Model file for the job. Use its own axes, mm. Coordinates: 2 decimals unless noted, no trailing zeros. Write each loop counter-clockwise with the first axis right and the second up, starting at its lowest first coordinate (ties: lowest second). Pieces come first, ordered by that corner, then holes. Notation, with made-up numbers: M 51.5,-28.5 L 67.5,-28.5 A14 ccw 67.5,-14.5 Z; hole C 45.5,40.25 d3. An arc over 180 degrees is marked long. One line per question, with ' | ' between items. Start each with the question number.
(1) Cut at B-B (y = 1.5). Count the separate pieces of the cut face and the enclosed holes in it, plus the area to 3 significant figures.
(2) Two-plate mould, pull along Z, no slides. Class faces 1 (the face through (0.733, 1.479, 99.997)), 2 (the face through (42.495, 1.479, -41.232)), 3 (the face through (1, 3, 1)): +Z half, -Z half, draft (parallel to the pull), parting line (faces both ways), or undercut.
(3) Cut at A-A (x = 38). Write the cut outline in (y, z), plus the area to 3 significant figures.
(4) Wall check: probe 1 along Z at (x, y) = (-25, 2.15); probe 2 along Z at (x, y) = (-41, 1.8); probe 3 along X at (y, z) = (0.55, 91.5). Give the ranges that are in metal, low to high.
(5) Flat gauge pin, fed straight in: pin 1 Ø3.5 at (x, z) = (-42, 84.85) entering from -Y. Where does the tip first touch, or does it go through?
(6) Cut at D-D (x = -17.5). Write the cut outline in (y, z).
(7) Cut at C-C (x = -37.5). Write the cut outline in (y, z), plus the area to 3 significant figures.
Autodesk Inventor part; units mm, degrees
ref_plane "YZ Plane" through (0, 0, 0) normal (1, 0, 0) x (0, 1, 0)
ref_plane "XZ Plane" through (0, 0, 0) normal (0, 1, 0) x (-1, 0, 0)
ref_plane "XY Plane" through (0, 0, 0) normal (0, 0, 1) x (1, 0, 0)
sketch "Sketch1" plane through (0, 0, 0) normal (0, 1, 0) x (-1, 0, 0)
  line L0 (-50, 86.6025) -> (-50, -86.6025)
  line L1 (50, -86.6025) -> (50, 86.6025)
  arc A0 (50, 86.6025) -> (-50, 86.6025) centre (0, 0) ccw
  arc A1 (-50, -86.6025) -> (50, -86.6025) centre (0, 0) ccw
  circle A2 centre (25, -67.0117) radius 1.35
  circle A3 centre (25, -9.0117) radius 1.35
  circle A4 centre (-24, -9.0117) radius 1.35
  circle A5 centre (-24, -67.0117) radius 1.35
  circle A6 centre (42, -84.8528) radius 1.3
  circle A7 centre (42, -60.6528) radius 1.3
  circle A8 centre (-42, -84.8528) radius 1.3
  circle A9 centre (-42, -60.6528) radius 1.3
  circle A10 centre (42, 84.8528) radius 1.3
  circle A11 centre (42, 60.6528) radius 1.3
  circle A12 centre (-42, 84.8528) radius 1.3
  circle A13 centre (-42, 60.6528) radius 1.3
  circle A14 centre (23.5943, 91.1005) radius 1.3
  circle A15 centre (-23.9057, 91.1005) radius 1.3
  circle A16 centre (37.5, -41.0117) radius 5
  circle A17 centre (-37.5, -41.0117) radius 5
extrude "Extrusion1" add sketch "Sketch1" along normal blind 3
properties part number "basePlate3"
Filled in:
1) separate pieces: 1 | enclosed holes: 16 | area: 18,900 mm²
2) face 1: +Z half | face 2: undercut | face 3: draft
3) outline: M 0,-92.5 L 3,-92.5 L 3,-45.99 L 0,-45.99 Z; M 0,-36.04 L 3,-36.04 L 3,92.5 L 0,92.5 Z | area: 525 mm²
4) probe 1: -96.82 to -68.36, -65.66 to -10.36, -7.66 to 96.82 | probe 2: -91.21 to -85.68, -84.02 to -61.48, -59.82 to -44.58, -37.44 to 59.82, 61.48 to 84.02, 85.68 to 91.21 | probe 3: -40.35 to -24.83, -22.36 to 22.67, 25.14 to 40.35
5) pin 1: y = 0
6) outline: M 0,-98.46 L 3,-98.46 L 3,98.46 L 0,98.46 Z
7) outline: M 0,-92.7 L 3,-92.7 L 3,-46.01 L 0,-46.01 Z; M 0,-36.01 L 3,-36.01 L 3,92.7 L 0,92.7 Z | area: 526 mm²
